Verification items for this drawing (mm, ordinates from the low corner). A direction names the side the tool comes from. Coordinates: 2 decimals unless noted, no trailing zeros. Order: outer loops, then holes, each group sorted by start corner. A loop starts at its lowest first (then second) coordinate and runs counter-clockwise, first axis right, second up. Notation, with made-up numbers: M 22,40 L 57,40 A9 ccw 57,48 Z; hole C -21,13 d11. An arc over 180 degrees is marked long. Write item = value, one per line.
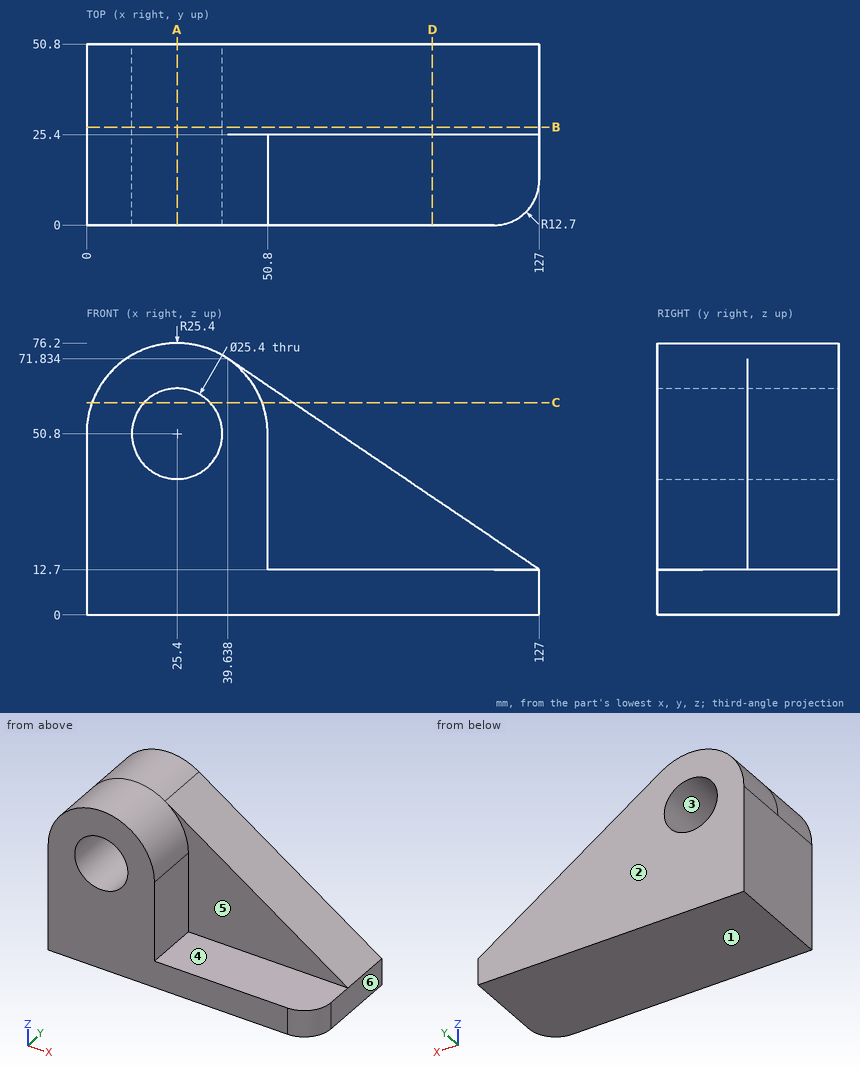
Item 1: Gauge pin test, flat ends, axial feed: pin 1 (1 mm diameter, centred on y = 43.5, z = 43.5, fed in from -X); pin 2 (1.5 mm diameter, centred on y = 26.5, z = 31, fed in from +X); pin 3 (1 mm diameter, centred on y = 8, z = 40.5, fed in from +X); pin 4 (4 mm diameter, centred on x = 66.5, z = 36.5, fed in from -Y). Record the tip position at first contact, or that the pin passes through.
Report:
pin_1 = 0
pin_2 = 101.07
pin_3 = 50.8
pin_4 = 25.4
Item 2: Sectioned sample at C-C, the plane z = 59.5. Enter the section's corners in (x, y), then the cut area to 3 significant figures.
Report:
outline = M 1.54,0 L 16.15,0 L 16.15,50.8 L 1.54,50.8 Z; M 34.65,0 L 49.26,0 L 49.26,25.4 L 57.86,25.4 L 57.86,50.8 L 34.65,50.8 Z
area = 1,700 mm^2
Item 3: Tool access check on the marked faces 5 and 6. Record the directions out of +Z, -Z, +X, -X, +Y, -Y that give a thin tool (end or side, any length) a straight path to the whole face; none if there is none.
Report:
face_5 = +Z, +X, -Y
face_6 = +Z, -Z, +X, +Y, -Y
Item 4: Sectioned sample at B-B, the plane y = 27.5. Enter the section's corners in (x, z), then the cut area to 3 significant figures.
Report:
outline = M 0,0 L 127,0 L 127,12.7 L 39.64,71.83 A25.4 ccw 0,50.8 Z; hole C 25.4,50.8 d25.4
area = 6,050 mm^2
Item 5: Release check for a two-part mould opening along Z. For the marked faces 1, 2, 3 and 4 record: pulls with the +Z half, pulls with the -Z half, needs draft (parallel to the pull), parting line crosses it, or undercut.
Report:
face_1 = pulls with the -Z half
face_2 = needs draft
face_3 = undercut
face_4 = pulls with the +Z half
Item 6: Scan lines: L1, parallel to Y at x = 111, z = 14; L2, parallel to X at y = 23.5, z = 37; L3, parallel to Z at x = 33.5, y = 8 (1 decimal). Record each from-to range of solid material in increasing order. Write a range as from..to.
Report:
L1 = 25.4..50.8
L2 = 0..50.8
L3 = 0..41, 60.6..74.9
Item 7: Sectioned sample at D-D, the plane x = 97. Enter the section's corners in (y, z).
Report:
outline = M 0,0 L 50.8,0 L 50.8,33.01 L 25.4,33.01 L 25.4,12.7 L 0,12.7 Z
Item 8: Sectioned sample at A-A, the plane x = 25.4. Enter the section's corners in (y, z), then the cut area to 3 significant figures.
Report:
outline = M 0,0 L 50.8,0 L 50.8,38.1 L 0,38.1 Z; M 0,63.5 L 50.8,63.5 L 50.8,76.2 L 0,76.2 Z
area = 2,580 mm^2
